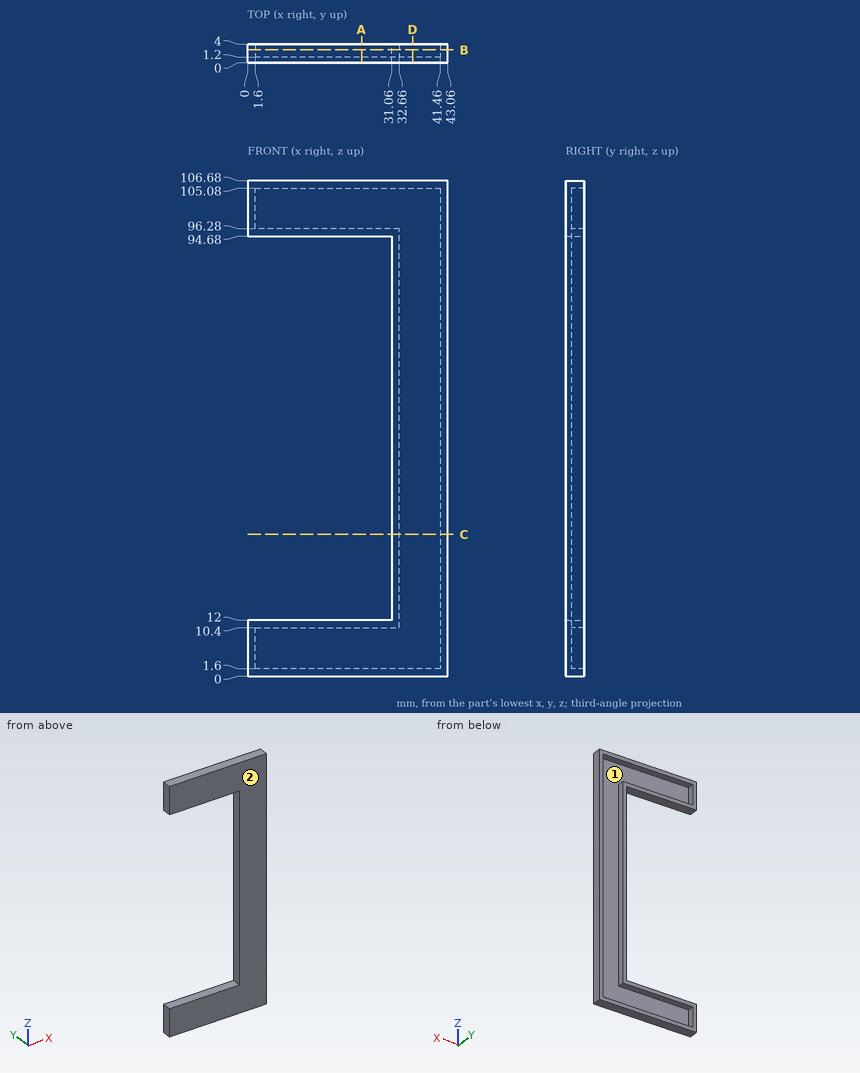
Study the drawing (mm; zero at the part's minimum x, y, z) and answer. Give positions to 0.01 mm unless a question says otherwise; leave off trailing zeros. Loops run counter-clockwise (first coordinate to the right, second up) from the corner with the lowest first, then second, coordinate; pieces in that order, holes last. Notation, with made-up numbers: (84.5, 42) - (137.5, 42) arc R10 cw to (137.5, 52) - close; hole circle Ø3 at (16, -35.5). An arc over 180 degrees is marked (long way). Use CSV: the item, a comma, the result in double quotes. Start each with the question number.
(1) Each of these flat-tipped pins is pushed along its axis until it touches: pin 1 (2 mm diameter, centred on x = 7.5, y = 2, fed in from -Z); pin 2 (2 mm diameter, centred on y = 3, z = 35, fed in from -X); pin 3 (12 mm diameter, centred on x = 23.5, z = 60, fed in from -Y); pin 4 (4 mm diameter, centred on x = 36.5, z = 71, fed in from +Y). Where does it stop, or does it pass through?
(2) Find section C-C, the plane z = 30.5. Determine the outline of the cut face in (x, y), plus the area to 3 significant figures.
(3) Find section D-D, the plane x = 35.5. Determine the outline of the cut face in (y, z).
(4) Determine the mould class of the marked faces 1 and 2 for opening direction X: released by +X, released by -X, zero draft, split by the parting line, or undercut.
(5) Find the intervals of material crossed by L1, parallel to Z at x = 2.5, y = 1.85; L2, parallel to X at y = 2.3, z = 93.5; L3, parallel to X at y = 0.6, z = 70.5, in increasing order.
(6) Find section A-A, the plane x = 24.5. Determine the outline of the cut face in (y, z), plus the area to 3 significant figures.
(7) Find section B-B, the plane y = 2.75. Determine the outline of the cut face in (x, z).
Results found:
1,pin 1,"z = 0"
1,pin 2,"x = 31.06"
1,pin 3,"through"
1,pin 4,"y = 1.2"
2,outline,"(31.06, 0) - (43.06, 0) - (43.06, 4) - (41.46, 4) - (41.46, 1.2) - (32.66, 1.2) - (32.66, 4) - (31.06, 4) - close"
2,area,"23.4 mm^2"
3,outline,"(0, 0) - (4, 0) - (4, 1.6) - (1.2, 1.6) - (1.2, 105.08) - (4, 105.08) - (4, 106.68) - (0, 106.68) - close"
4,face 1,"undercut"
4,face 2,"zero draft"
5,L1,"0 to 1.6, 10.4 to 12, 94.68 to 96.28, 105.08 to 106.68"
5,L2,"31.06 to 32.66, 41.46 to 43.06"
5,L3,"31.06 to 43.06"
6,outline,"(0, 0) - (4, 0) - (4, 1.6) - (1.2, 1.6) - (1.2, 10.4) - (4, 10.4) - (4, 12) - (0, 12) - close; (0, 94.68) - (4, 94.68) - (4, 96.28) - (1.2, 96.28) - (1.2, 105.08) - (4, 105.08) - (4, 106.68) - (0, 106.68) - close"
6,area,"46.7 mm^2"
7,outline,"(0, 0) - (43.06, 0) - (43.06, 106.68) - (0, 106.68) - (0, 94.68) - (31.06, 94.68) - (31.06, 12) - (0, 12) - close; hole (1.6, 1.6) - (41.46, 1.6) - (41.46, 105.08) - (1.6, 105.08) - (1.6, 96.28) - (32.66, 96.28) - (32.66, 10.4) - (1.6, 10.4) - close"
